Design review of the part built by this model. Coordinates are the model's own, in mm. A direction names the side the tool comes from. Give positions to 0.01 mm unless a question says otherwise; leave off trailing zeros. Order: outer loops, then holes, each group sorted by start corner. A loop starts at its lowest first (then second) coordinate and runs counter-clockwise, first axis right, second up.
Autodesk Inventor part; units mm, degrees
ref_plane "Work Plane3" through (3.9126, 0, 0) normal (1, 0, 0) x (0, 1, 0)
ref_plane "XZ Plane" through (0, 0, 0) normal (0, 1, 0) x (-1, 0, 0)
ref_plane "XY Plane" through (0, 0, 0) normal (0, 0, 1) x (1, 0, 0)
sketch "Sketch1" plane through (0, 0, 0) normal (0, 0, 1) x (1, 0, 0)
  line L0 (0, 0) -> (-8.052, 0) construction
  line L1 (-6.096, 2.032) -> (5.08, 2.032)
  line L2 (-6.096, 2.032) -> (-6.096, 3.2258)
  line L3 (-6.096, 3.2258) -> (0, 3.2258)
  line L4 (0, 3.2258) -> (0, 6.9215)
  line L5 (0, 6.9215) -> (-3.81, 6.9215)
  line L6 (-3.81, 6.9215) -> (-3.81, 13.5001)
  line L7 (-3.81, 13.5001) -> (0, 13.5001)
  arc A0 (5.08, 2.032) -> (0, 13.5001) centre (-14.9919, 0) ccw
  dimension "d0" = 2.032
  dimension "d1" = 13.5001
  dimension "d2" = 6.096
  dimension "d3" = 3.2258
  dimension "d4" = 3.81
  dimension "d5" = 6.9215
  dimension "d7" = 5.08
revolve "Revolution1" add sketch "Sketch1" angle 360 about axis through (0, 0, 0) along (-1, 0, 0)
ref_plane "Work Plane3" through (3.9126, 0, 0) normal (1, 0, 0) x (0, 1, 0)
ref_plane "Work Plane2" through (5.1826, 0, 0) normal (1, 0, 0) x (0, 1, 0)
sketch "Sketch2" plane through (3.9126, 0, 0) normal (1, 0, 0) x (0, 1, 0)
  circle A0 centre (0, 0) radius 2.032
  line L0 (-1.6801, -1.143) -> (1.6801, -1.143)
  dimension "d10" = 3.175
extrude "Extrusion1" add sketch "Sketch2" against normal blind 6.604 contours L0 A0 picked at (-0.4517, -1.2667)
sketch "Sketch3" plane through (-2.6914, 0, 0) normal (-1, 0, 0) x (0, 0, 1)
  arc A0 (-1.143, 1.6801) -> (-1.143, -1.6801) centre (0, 0) ccw
  line L0 (-1.143, -1.6801) -> (-1.143, 1.6801)
  circle A1 centre (0, 0) radius 1.143
  circle A2 centre (0, 0) radius 2.032
  dimension "d13" = 2.286
extrude "Extrusion2" add sketch "Sketch3" along normal up to surface (3.4046 mm away)
sketch "Sketch4" plane through (-3.81, 0, 0) normal (-1, 0, 0) x (0, 0, 1)
  circle A0 centre (0, 10.16) radius 1.7272
extrude "Extrusion3" cut sketch "Sketch4" against normal through all
chamfer "Chamfer1" distance 0.762 angle 45 4 edges at (-3.81, -13.5001, 0) (-3.81, -6.9215, 0) (-6.096, -3.2258, 0) (-6.096, 0, -1.143)
sketch "Sketch5" plane through (3.9126, 0, 0) normal (1, 0, 0) x (0, 1, 0)
  circle A0 centre (0, 0) radius 22.931
extrude "Extrusion4" cut sketch "Sketch5" along normal blind 25.4
properties part number "Flexiwheel Hub - Motor Side"
1. Take a section at A-A (x = -4.25). State the section outline as (y, z) points.
Recorded:
outline: circle Ø6.45 at (0, 0); hole circle Ø2.29 at (0, 0)
2. Machinability: for faces 4 (the face through (-2.691, -1, 1)), 5 (the face through (-1.081, 8.474, -0.374)), 6 (the face through (-1.545, 3.721, -5.836)), which of the approach directions +Z, -Z, +X, -X, +Y, -Y give a long, thin tool a straight path to every point of the face, cutting with its end or side? Answer none if there is none.
Recorded:
face 4: +X
face 5: +X, -X
face 6: -X
3. For pin 1 (5 mm diameter, centred on y = 11, z = -3, fed in from +X); pin 2 (4 mm diameter, centred on y = -7.5, z = 9.5, fed in from +X); pin 3 (2.5 mm diameter, centred on y = 0, z = 0, fed in from -X); pin 4 (1 mm diameter, centred on y = 0.5, z = 0, fed in from +X), all flat-tipped, find the tip position at first contact; note any pin that passes through.
Recorded:
pin 1: stops at x = 3.11
pin 2: stops at x = 2.47
pin 3: stops at x = -5.44
pin 4: passes through
4. Take a section at B-B (z = 0). State how many separate pieces and enclosed holes the cut face has, then the cut area to 3 significant figures.
Recorded:
separate pieces: 3
enclosed holes: 0
area: 115 mm2
5. Draft analysis for pull direction Z (two halves, no side actions). For faces 1 (the face through (-1.503, -10.713, -8.215)), 2 (the face through (-6.096, 1, 2)), 3 (the face through (-2.63, 3.077, 0.969)), state which applies: pulls with the +Z half, pulls with the -Z half, needs draft (parallel to the pull), parting line crosses it, or undercut.
Recorded:
face 1: parting line crosses it
face 2: needs draft
face 3: undercut
6. For line 1 along Y through (x, z) = (-1.3, 0); line 2 along Y through (x, z) = (-2.25, 2.75); line 3 along Y through (x, z) = (-3.5, 0), list the stretches that pass through material, from the lowest coordinate up.
Recorded:
line 1: y = -13.5 to -6.92, -3.23 to -2.03, 2.03 to 3.23, 6.92 to 8.43, 11.89 to 13.5
line 2: y = -13.22 to -6.35, -1.69 to 1.69, 6.35 to 13.22
line 3: y = -13.05 to -7.37, -3.23 to -1.14, 1.14 to 3.23, 7.37 to 8.43, 11.89 to 13.05
